```python
from build123d import *

# Parameters (mm, degrees)
F1_R      = 1.35
F7_DEPTH  = 10
F6_R      = 1.35
F8_DEPTH  = 10
F9_R      = 25.5937233364
F10_DEPTH = 32.8702228284


with BuildPart() as f5:
    # F0 (on Front) → F5 section 0
    with BuildSketch(Plane.XZ):
        with BuildLine():
            ThreePointArc((32.5, 27.5), (31.0355339059, 31.0355339059), (27.5, 32.5))
            Line((27.5, 32.5), (-27.5, 32.5))
            ThreePointArc((-27.5, 32.5), (-31.0355339059, 31.0355339059), (-32.5, 27.5))
            Line((-32.5, 27.5), (-32.5, -27.5))
            ThreePointArc((-32.5, -27.5), (-31.0355339059, -31.0355339059), (-27.5, -32.5))
            Line((-27.5, -32.5), (27.5, -32.5))
            ThreePointArc((27.5, -32.5), (31.0355339059, -31.0355339059), (32.5, -27.5))
            Line((32.5, -27.5), (32.5, 27.5))
        make_face()
    # F4 (on line) → F5 section 1
    with BuildSketch(Plane(origin=(0, -20.4416673649, 7.4401584596), x_dir=(-1, 0, 0), z_dir=(0, 0.9396926208, -0.3420201433))):
        with BuildLine():
            Line((27.5, 30.5400101755), (-27.5, 30.5400101755))
            add(Edge.make_bspline(
                [(-27.5, 30.5400101755), (-32.5, 30.5400101755), (-32.5, 25.8415470716)],
                knots=[4.7123889804, 4.7123889804, 4.7123889804, 6.2831853072, 6.2831853072, 6.2831853072], degree=2, weights=[1, 0.7071067812, 1]))
            Line((-32.5, 25.8415470716), (-32.5, -25.8415470716))
            add(Edge.make_bspline(
                [(-32.5, -25.8415470716), (-32.5, -30.5400101755), (-27.5, -30.5400101755)],
                knots=[0, 0, 0, 1.5707963268, 1.5707963268, 1.5707963268], degree=2, weights=[1, 0.7071067812, 1]))
            Line((-27.5, -30.5400101755), (27.5, -30.5400101755))
            add(Edge.make_bspline(
                [(27.5, -30.5400101755), (32.5, -30.5400101755), (32.5, -25.8415470716)],
                knots=[1.5707963268, 1.5707963268, 1.5707963268, 3.1415926536, 3.1415926536, 3.1415926536], degree=2, weights=[1, 0.7071067812, 1]))
            Line((32.5, -25.8415470716), (32.5, 25.8415470716))
            add(Edge.make_bspline(
                [(32.5, 25.8415470716), (32.5, 30.5400101755), (27.5, 30.5400101755)],
                knots=[3.1415926536, 3.1415926536, 3.1415926536, 4.7123889804, 4.7123889804, 4.7123889804], degree=2, weights=[1, 0.7071067812, 1]))
        make_face()
    loft()

    # F1 (on Front) → F7 (cut)
    with BuildSketch(Plane.XZ):
        with Locations((-25, 25)):
            Circle(F1_R)
        with Locations((25, 25)):
            Circle(F1_R)
        with Locations((-25, -25)):
            Circle(F1_R)
        with Locations((25, -25)):
            Circle(F1_R)
    extrude(amount=F7_DEPTH, mode=Mode.SUBTRACT)

    # F6 (on line) → F8 (cut)
    with BuildSketch(Plane(origin=(0, -20.4416673649, 7.4401584596), x_dir=(-1, 0, 0), z_dir=(0, 0.9396926208, -0.3420201433))):
        with Locations((-25, 25)):
            Circle(F6_R)
        with Locations((25, 25)):
            Circle(F6_R)
        with Locations((-25, -25)):
            Circle(F6_R)
        with Locations((25, -25)):
            Circle(F6_R)
    extrude(amount=F8_DEPTH, mode=Mode.SUBTRACT)

    # F9 (on face) → F10 (cut, through all)
    with BuildSketch(Plane(origin=(0, -20.4416673649, 7.4401584596), x_dir=(1, 0, 0), z_dir=(0, -0.9396926208, 0.3420201433))):
        Circle(F9_R)
    extrude(amount=-F10_DEPTH, mode=Mode.SUBTRACT)


solid = f5.part
```
Could you check a few things on this model? Use its own coordinates, in mm. A direction names the side the tool comes from. Give positions to 0.01 mm unless a question says otherwise; leave off trailing zeros. Loops run counter-clockwise (first coordinate to the right, second up) from the corner with the lowest first, then second, coordinate; pieces in that order, holes last. Notation, with made-up numbers: (83, 50) - (87, 50) arc R10 ccw to (87, 63) - close; hole circle Ø3 at (52.5, -4). An arc over 180 degrees is marked (long way). Answer in a Markdown table with one row per item. Add a question column.
Q1. If we section it at A-A (x = 22): List the corners of the cut face in (y, z) for me.
Q2. Which directions (+Z, -Z, +X, -X, +Y, -Y) give clear straight access to the entire face, cutting with the end or side of a thin tool? Please do faces 4 (the face through (0.385, -5.068, 34.345)), 5 (the face through (-24.981, -19.589, -19.455)), 6 (the face through (25, -10, 25)).
Q3. For pin 1 (0.8 mm diameter, centred on x = -25, z = -25.5, fed in from +Y); pin 2 (12 mm diameter, centred on x = -9.5, z = -4, fed in from -Y); pin 3 (3 mm diameter, centred on x = 3, y = -13, fed in from -Z); pin 4 (2 mm diameter, centred on x = -25, z = 25, fed in from -Y), each with a flat end and sliding along its axis, tell me the tip position at first contact or that it passes through.
Q4. We'd pull the mould along Z, two halves only. Please class faces 1 (the face through (-25.46, -18.13, 13.79)), 2 (the face through (23.753, -7.435, 28.76)), 3 (the face through (-22, 0, 15)): +Z half, -Z half, draft (parallel to the pull), parting line (faces both ways), or undercut.
Q5. If we section it at B-B (x = -17): List the corners of the cut face in (y, z) for me, plus the area to 3 significant figures.
Q6. Please list where these lines run through material, in increasing order: L1, parallel to Y at x = -23, z = -12; L2, parallel to X at y = -4, z = 24; L3, parallel to X at y = -9, z = -12.5. Write a range as from..to.
The answers:
| question | item | result |
|---|---|---|
| 1 | outline | (-30.89, -21.26) - (0, -32.5) - (0, -13.92) - (-24.91, -4.85) - close; (-15.97, 19.73) - (0, 13.92) - (0, 32.5) - (-10, 36.14) - close |
| 2 | face 4 | +Z, +X, -X, +Y |
| 2 | face 5 | none |
| 2 | face 6 | +Y |
| 3 | pin 1 | stops at y = -10 |
| 3 | pin 2 | passes through |
| 3 | pin 3 | stops at z = -28.31 |
| 3 | pin 4 | stops at y = -14.41 |
| 4 | face 1 | +Z half |
| 4 | face 2 | undercut |
| 4 | face 3 | draft |
| 5 | outline | (-30.89, -21.26) - (0, -32.5) - (0, -20.36) - (-26.99, -10.54) - close; (-13.9, 25.42) - (0, 20.36) - (0, 32.5) - (-10, 36.14) - close |
| 5 | area | 496 mm^2 |
| 6 | L1 | y = -27.52..0 |
| 6 | L2 | x = -32.5..-25.91, -24.09..-14.36, 14.36..24.09, 25.91..32.5 |
| 6 | L3 | x = -32.5..-20.86, 20.86..32.5 |
